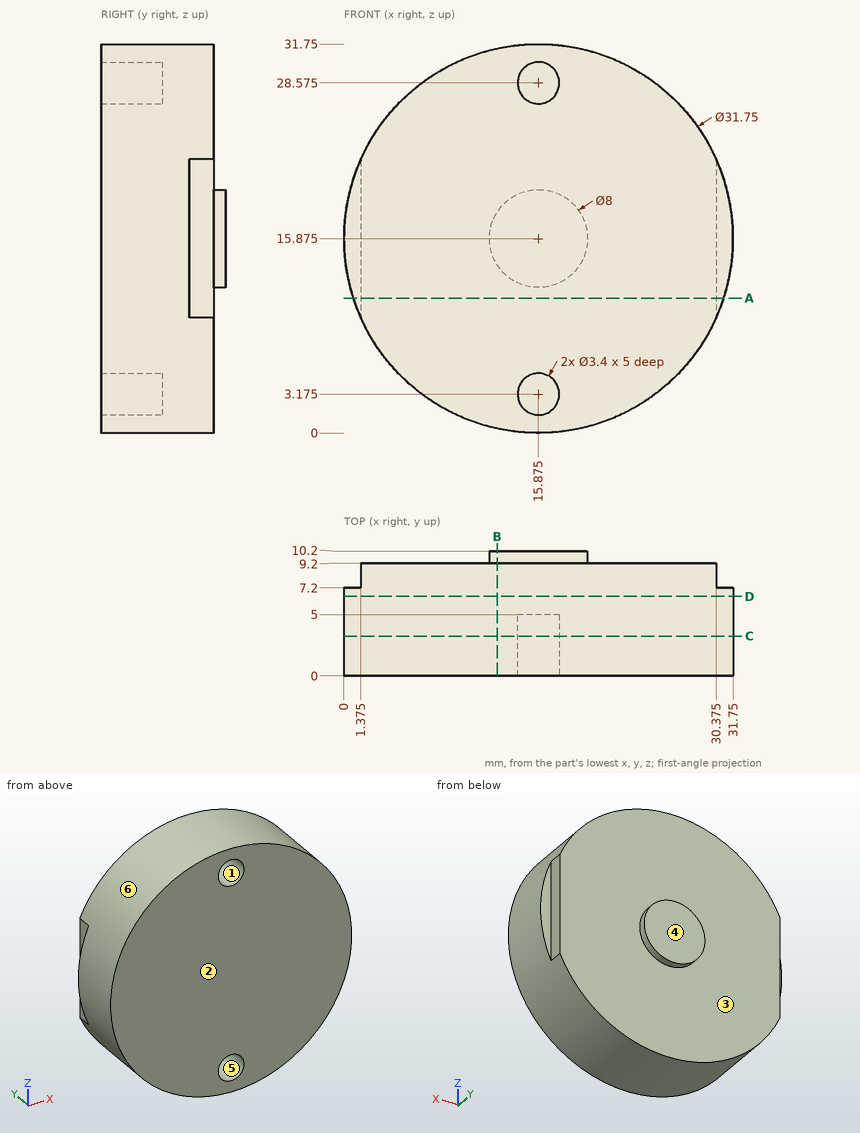
Answer from the drawing. Dimensions are ordinates in mm from the lowest x, y and z of the part. A direction names the side the tool comes from. Give positions to 0.01 mm unless a question says otherwise; leave off trailing zeros. Write each loop counter-clockwise with the first axis right and the second up, starting at its lowest first coordinate (ties: lowest second). Pieces come first, ordered by that corner, then holes. Notation, with made-up numbers: (58.25, 54) - (103.25, 54) arc R18 cw to (103.25, 70) - close; hole circle Ø9 at (83.25, 54). An arc over 180 degrees is marked (long way). One line per item, written item: value. Start each with the question number.
1. For the marked faces 1, 2 and 3, determine the directions among +Z, -Z, +X, -X, +Y, -Y from which every point of the face is accessible in a straight line to the end or side of a thin tool.
2. Consider probe 1 along Y at (x, z) = (4.5, 10); probe 2 along Y at (x, z) = (17, 28.5); probe 3 along X at (y, z) = (4.25, 11). Determine where each line is inside the solid, lowest interval first.
3. For a pull along Z with two mould halves and no side action, classify the marked faces 4, 5 and 6 as +Z half, -Z half, draft (parallel to the pull), parting line (faces both ways), or undercut.
4. Find section D-D (y = 6.5). Write down the section's boundary in (x, z) (3 decimals).
5. Find section C-C (y = 3.25). Write down the section's boundary in (x, z) (3 decimals), then the cut area to 3 significant figures.
6. Find section A-A (z = 11). Write down the section's boundary in (x, y) (3 decimals), then the cut area to 3 significant figures.
7. Given pin 1 (2.5 mm diameter, centred on x = 16.5, z = 28, fed in from -Y); pin 2 (3 mm diameter, centred on x = 6, z = 15, fed in from +Y); pin 3 (2 mm diameter, centred on x = 17.5, y = 2.5, fed in from -Z); pin 4 (1 mm diameter, centred on x = 23.5, y = 3, fed in from -Z), each flat-ended and moving along its own axis, determine where each tip first touches the part or whether it passes through.
8. Find section B-B (x = 12.5). Write down the section's boundary in (y, z).
Geometry results:
1. face 1: -Y
1. face 2: +Z, -Z, +X, -X, -Y
1. face 3: +Y
2. probe 1: 0 to 9.2
2. probe 2: 5 to 9.2
2. probe 3: 0.77 to 30.98
3. face 4: draft
3. face 5: undercut
3. face 6: parting line
4. outline: circle Ø31.75 at (15.875, 15.875)
5. outline: circle Ø31.75 at (15.875, 15.875); hole circle Ø3.4 at (15.875, 3.175); hole circle Ø3.4 at (15.875, 28.575)
5. area: 774 mm2
6. outline: (0.767, 0) - (30.983, 0) - (30.983, 7.2) - (30.375, 7.2) - (30.375, 9.2) - (1.375, 9.2) - (1.375, 7.2) - (0.767, 7.2) - close
6. area: 276 mm2
7. pin 1: y = 0
7. pin 2: y = 9.2
7. pin 3: z = 0.01
7. pin 4: z = 1.69
8. outline: (0, 0.36) - (9.2, 0.36) - (9.2, 13.73) - (10.2, 13.73) - (10.2, 18.02) - (9.2, 18.02) - (9.2, 31.39) - (0, 31.39) - close
